Design review of the part built by this model. Coordinates are the model's own, in mm. A direction names the side the tool comes from. Give positions to 0.01 mm unless a question says otherwise; leave off trailing zeros. Order: outer loops, then holes, each group sorted by start corner. A loop starts at its lowest first (then second) coordinate and runs counter-clockwise, first axis right, second up. Notation, with made-up numbers: (-0.75, -12) -> (11.25, -12) arc R8 ccw to (11.25, 0) -> close; hole circle Ø9 at (0, 0). An arc over 180 degrees is marked (long way). One line per item, written item: value. Start each with the question number.
1) Consider section A-A (z = 45). State the section outline as (x, y) points, plus the area to 3 significant figures.
2) Consider section B-B (y = 11.5). State the section outline as (x, z) points, plus the area to 3 significant figures.
3) Consider section D-D (z = 12). State the section outline as (x, y) points.
4) Tool access review of faces 1 (the face through (-4.507, -4.213, 35.161)), 2 (the face through (0, -14, 25)), 3 (the face through (0, 15, 25)): name each direction out of +Z, -Z, +X, -X, +Y, -Y from which nothing blocks a thin tool from reaching the whole face with its end or side.
5) Wall thickness on line 1 along X through (y, z) = (-14.6, 45); line 2 along X through (y, z) = (5.75, 13.5); line 3 along Y through (x, z) = (0.25, 37.5): over which ranges is each line inside the solid? List them lowest first. Write a range as from..to.
6) Consider section C-C (x = 2.5). State the section outline as (y, z) points.
7) The part is to be moulded in two halves that separate along Z. For faces 4 (the face through (1.08, 14.51, 43.82)), 5 (the face through (0, 14, 25)), 6 (the face through (-4.5, 1.2, 0)), say which applies: released by +Z, released by -Z, zero draft, split by the parting line, or undercut.
from build123d import *

# Parameters (mm, degrees)
SKETCH_289_W           = 10
SKETCH_289_H           = 30
SKETCH_289_W_2         = 8
SKETCH_289_H_2         = 28
EXTRUDE_359_DEPTH      = 50
SKETCH_433_R           = 1.6
CUT_EXTRUDE_966_DEPTH  = 59.523499554
SKETCH_661_R           = 9.5
CUT_EXTRUDE_1010_DEPTH = 54.150729064
CUT_EXTRUDE_1_REACH    = 55.151
SKETCH_1_R             = 11


with BuildPart() as part:
    # Sketch 289 → Extrude 359 (new body)
    with BuildSketch(Plane.XY):
        Rectangle(SKETCH_289_W, SKETCH_289_H)
        Rectangle(SKETCH_289_W_2, SKETCH_289_H_2, mode=Mode.SUBTRACT)
    extrude(amount=EXTRUDE_359_DEPTH)

    # Sketch 433 → Cut-Extrude 966 (cut, through all)
    with BuildSketch(Plane(origin=(0, 15, 0), x_dir=(1, 0, 0), z_dir=(0, 1, 0))):
        with Locations(Location((0, -5, 0), (0, 0, 270))):
            Circle(SKETCH_433_R)
        with Locations(Location((0, -45, 0), (0, 0, 270))):
            Circle(SKETCH_433_R)
    extrude(amount=-CUT_EXTRUDE_966_DEPTH, mode=Mode.SUBTRACT)

    # Sketch 661 → Cut-Extrude 1010 (cut, through all)
    with BuildSketch(Plane(origin=(5, 0, 0), x_dir=(0, 0, -1), z_dir=(1, 0, 0))):
        with Locations((-25, 0)):
            Circle(SKETCH_661_R)
    extrude(amount=-CUT_EXTRUDE_1010_DEPTH, mode=Mode.SUBTRACT)

    # ｽｹｯﾁ1 → ｶｯﾄ - 押し出し1 (cut, up to next)
    with BuildSketch(Plane.ZY.offset(5), mode=Mode.PRIVATE) as cut_extrude_1_sk1:
        with Locations((25, 0)):
            Circle(SKETCH_1_R)
    cut_extrude_1_tool1 = extrude(cut_extrude_1_sk1.sketch, amount=-CUT_EXTRUDE_1_REACH, mode=Mode.PRIVATE) & part.part
    add(cut_extrude_1_tool1.solids().sort_by_distance((-5, 0, 25))[0], mode=Mode.SUBTRACT)


solid = part.part
Checked values:
1. outline: (-5, -15) -> (-1.6, -15) -> (-1.6, -14) -> (-4, -14) -> (-4, 14) -> (-1.6, 14) -> (-1.6, 15) -> (-5, 15) -> close; (1.6, -15) -> (5, -15) -> (5, 15) -> (1.6, 15) -> (1.6, 14) -> (4, 14) -> (4, -14) -> (1.6, -14) -> close
1. area: 69.6 mm^2
2. outline: (-5, 0) -> (-4, 0) -> (-4, 50) -> (-5, 50) -> close; (4, 0) -> (5, 0) -> (5, 50) -> (4, 50) -> close
2. area: 100 mm^2
3. outline: (-5, -15) -> (5, -15) -> (5, 15) -> (-5, 15) -> close; hole (-4, -14) -> (4, -14) -> (4, 14) -> (-4, 14) -> close
4. face 1: -X
4. face 2: +Z, -Z
4. face 3: +Z, -Z, +X, -X, +Y
5. line 1: x = -5..-1.6, 1.6..5
5. line 2: x = -5..-4, 4..5
5. line 3: y = -15..-14, 14..15
6. outline: (-15, 0) -> (-14, 0) -> (-14, 50) -> (-15, 50) -> close; (14, 0) -> (15, 0) -> (15, 50) -> (14, 50) -> close
7. face 4: undercut
7. face 5: zero draft
7. face 6: released by -Z
